Geometry: final body of the model. Coordinates: model frame, mm. A direction names the side the tool comes from. Round coordinates to 2 decimals unless told otherwise and drop trailing zeros. Loops run counter-clockwise (first coordinate to the right, second up) from the corner with the lowest first, then second, coordinate; pieces in that order, holes last. Notation, with made-up numbers: (-31, 51.5) - (-19, 51.5) arc R14 ccw to (-19, 57.5) - close; hole circle Ø11 at (58, -38.5). An arc over 180 degrees is marked (long way). Answer as CSV lines item,"result".
from build123d import *

# Parameters (mm, degrees)
EXTRUDE_1_OUTLINE_R   = 90
EXTRUDE_1_OUTLINE_R_2 = 2
EXTRUDE_1_DEPTH       = 3
SKETCH_4_W            = 10.552817488
SKETCH_4_H            = 70.751844526
EXTRUDE_2_DEPTH       = 30
CUT_EXTRUDE_1_DEPTH   = 30


# Read off the part's stored shape, not the designer's step: 填料-伸長1
with BuildPart() as part:
    # 填料-伸長1 outline → 填料-伸長1 (new body)
    with BuildSketch(Plane.XY):
        Circle(EXTRUDE_1_OUTLINE_R)
        with Locations((-60, -55)):
            Circle(EXTRUDE_1_OUTLINE_R_2, mode=Mode.SUBTRACT)
        with Locations((60, -55)):
            Circle(EXTRUDE_1_OUTLINE_R_2, mode=Mode.SUBTRACT)
        with Locations((-60, 55)):
            Circle(EXTRUDE_1_OUTLINE_R_2, mode=Mode.SUBTRACT)
        with Locations((60, 55)):
            Circle(EXTRUDE_1_OUTLINE_R_2, mode=Mode.SUBTRACT)
    extrude(amount=EXTRUDE_1_DEPTH)

    # 草圖4 → 填料-伸長2 (add)
    with BuildSketch(Plane(origin=(0, 0, 3), x_dir=(-1, 0, 0), z_dir=(0, 0, -1))):
        with Locations((71.471354809, 0)):
            Rectangle(SKETCH_4_W, SKETCH_4_H)
    extrude(amount=-EXTRUDE_2_DEPTH)

    # 草圖5 → 除料-伸長1 (cut)
    with BuildSketch(Plane.XY.offset(3)):
        with BuildLine():
            Line((68.5, -40), (71.5, -40))
            ThreePointArc((71.5, -40), (72.207106781, -39.707106781), (72.5, -39))
            Line((72.5, -39), (72.5, 39))
            ThreePointArc((72.5, 39), (72.207106781, 39.707106781), (71.5, 40))
            Line((71.5, 40), (68.5, 40))
            ThreePointArc((68.5, 40), (67.792893219, 39.707106781), (67.5, 39))
            Line((67.5, 39), (67.5, -39))
            ThreePointArc((67.5, -39), (67.792893219, -39.707106781), (68.5, -40))
        make_face()
    extrude(amount=-CUT_EXTRUDE_1_DEPTH, mode=Mode.SUBTRACT)


solid = part.part
(1) Section C-C (z = 13.5). Output: boundary loops of the cut face in (x, y).
Findings below:
outline,"(-76.75, -35.38) - (-66.19, -35.38) - (-66.19, 35.38) - (-76.75, 35.38) - close"
(2) Access query for faces 1 (the face through (-71, 35.376, 18)), 2 (the face through (-66.195, 0, 18)), 3 (the face through (-71, -35.376, 18)). Directions: +Z, -Z, +X, -X, +Y, -Y. A direction counts if a zero-diameter tool reaches every point of the face in a straight line with its end or side. Return the directions, or none.
Findings below:
face 1,"+Z, +X, -X, +Y"
face 2,"+Z, +X, +Y, -Y"
face 3,"+Z, +X, -X, -Y"
(3) Section D-D (y = -14.5). Output: boundary loops of the cut face in (x, z), and give its area (3 significant figures).
Findings below:
outline,"(-88.82, 0) - (67.5, 0) - (67.5, 3) - (-66.19, 3) - (-66.19, 33) - (-76.75, 33) - (-76.75, 3) - (-88.82, 3) - close; (72.5, 0) - (88.82, 0) - (88.82, 3) - (72.5, 3) - close"
area,"835 mm2"
(4) Section A-A (y = 30). Output: boundary loops of the cut face in (x, z), and give its area (3 significant figures).
Findings below:
outline,"(-84.85, 0) - (67.5, 0) - (67.5, 3) - (-66.19, 3) - (-66.19, 33) - (-76.75, 33) - (-76.75, 3) - (-84.85, 3) - close; (72.5, 0) - (84.85, 0) - (84.85, 3) - (72.5, 3) - close"
area,"811 mm2"
(5) Draft query along X for faces 4 (the face through (-71, 0, 33)), 5 (the face through (60, 57, 1)), 6 (the face through (-76.748, 0, 18)). Return one class per face: pulls with the +X half, pulls with the -X half, needs draft (parallel to the pull), parting line crosses it, or undercut.
Findings below:
face 4,"needs draft"
face 5,"undercut"
face 6,"pulls with the -X half"
(6) Material intervals for line 1 along Y through (x, z) = (-60, 0.9); line 2 along Z through (x, y) = (67, -41.5); line 3 along X through (y, z) = (-33.5, 24), sorted ascending.
Findings below:
line 1,"-67.08 to -57, -53 to 53, 57 to 67.08"
line 2,"0 to 3"
line 3,"-76.75 to -66.19"
(7) Section B-B (x = -54). Output: boundary loops of the cut face in (y, z), and give its area (3 significant figures).
Findings below:
outline,"(-72, 0) - (72, 0) - (72, 3) - (-72, 3) - close"
area,"432 mm2"
(8) Pin query (flat end, axial travel): P1, Ø3, axis at x = -71, z = 17.5, coming from the +Y side; P2, Ø8, axis at x = 53.5, y = -19.5, coming from the +Z side; P3, Ø2.5, axis at x = 70.5, z = 2, coming from the +Y side. Return the tip coordinate at first contact, or that it passes through.
Findings below:
P1,"y = 35.38"
P2,"z = 3"
P3,"y = 57.48"
